from build123d import *

# Parameters (mm, degrees)
F1_DEPTH = 31.75
F2_R     = 12.7
F4_DEPTH = 76.201


with BuildPart() as f1:
    # F0 (on Front) → F1 (new body)
    with BuildSketch(Plane.XZ):
        with BuildLine():
            ThreePointArc((-73.025, 0), (0, 73.025), (73.025, 0))
            Line((73.025, 0), (73.025, -73.025))
            Line((73.025, -73.025), (76.2, -73.025))
            Line((76.2, -73.025), (76.2, 0))
            ThreePointArc((76.2, 0), (0, 76.2), (-76.2, 0))
            Line((-76.2, 0), (-76.2, -73.025))
            Line((-76.2, -73.025), (-73.025, -73.025))
            Line((-73.025, -73.025), (-73.025, 0))
        make_face()
    extrude(amount=F1_DEPTH)

    # F2
    f2_edges = [f1.edges().sort_by_distance(p)[0] for p in [
        (-74.6125, -31.75, -73.025),
        (-74.6125, 0, -73.025),
        (74.6125, -31.75, -73.025),
        (74.6125, 0, -73.025),
    ]]
    fillet(f2_edges, radius=F2_R)

    # F3 (on Top) → F4 (cut, through all)
    with BuildSketch(Plane.XY):
        with BuildLine():
            ThreePointArc((-69.85, -17.4625), (-68.920064, -19.707564), (-66.675, -20.6375))
            Line((-66.675, -20.6375), (66.675, -20.6375))
            ThreePointArc((66.675, -20.6375), (68.920064, -19.707564), (69.85, -17.4625))
            Line((69.85, -17.4625), (69.85, -14.2875))
            ThreePointArc((69.85, -14.2875), (68.920064, -12.042436), (66.675, -11.1125))
            Line((66.675, -11.1125), (-66.675, -11.1125))
            ThreePointArc((-66.675, -11.1125), (-68.920064, -12.042436), (-69.85, -14.2875))
            Line((-69.85, -14.2875), (-69.85, -17.4625))
        make_face()
    extrude(amount=F4_DEPTH, mode=Mode.SUBTRACT)


solid = f1.part
Geometry: final body of the model. Coordinates: model frame, mm. A direction names the side the tool comes from. Give positions to 0.01 mm unless a question says otherwise; leave off trailing zeros. Loops run counter-clockwise (first coordinate to the right, second up) from the corner with the lowest first, then second, coordinate; pieces in that order, holes last. Notation, with made-up numbers: (44.5, -21) - (71.5, -21) arc R14 ccw to (71.5, 2) - close; hole circle Ø3 at (36, -10). An arc over 180 degrees is marked (long way). Answer as CSV lines item,"result". Start each with the question number.
1. Section D-D, the plane y = -2.5. Return loops of the section in (x, z) (3 decimals), plus the area to 3 significant figures.
2. Draft query along X for faces 1 (the face through (73.025, -16, -36)), 2 (the face through (1.68, -8.6, 76.18)), 3 (the face through (-74.59, -27.931, -69.403)). Return one class per face: released by +X, released by -X, zero draft, split by the parting line, or undercut.
3. Ray query, L1, parallel to X at y = -19.5, z = -18 (3 decimals); L2, parallel to Z at x = -1.5, y = -30; L3, parallel to X at y = -14.5, z = 5. Return the intervals inside material, ascending.
4. Section B-B, the plane z = -23. Return loops of the section in (x, y) (3 decimals), plus the area to 3 significant figures.
5. Reachability of faces 4 (the face through (74.635, -3.819, -69.403)), 5 (the face through (-73.025, -16, -37)) from +Z, -Z, +X, -X, +Y, -Y: full face, straight path, thin tool, end or side. Return the list, or none.
6. Section C-C, the plane z = 46. Return loops of the section in (x, y), plus the area to 3 significant figures.
7. Pin query (flat end, axial travel): P1, Ø3.5, axis at y = -16.5, z = 23.5, coming from the +X side; P2, Ø1, axis at x = 29, y = -8, coming from the -Z side; P3, Ø6, axis at x = -8, y = -9.5, coming from the +Z side. Return the tip coordinate at first contact, or that it passes through.
Answers:
1,outline,"(-76.2, -67.891) - (-73.025, -67.891) - (-73.025, 0) arc R73.025 cw to (73.025, 0) - (73.025, -67.891) - (76.2, -67.891) - (76.2, 0) arc R76.2 ccw to (-76.2, 0) - close"
1,area,"1,180 mm2"
2,face 1,"undercut"
2,face 2,"split by the parting line"
2,face 3,"zero draft"
3,L1,"x = -76.2 to -73.025, 73.025 to 76.2"
3,L2,"z = 73.01 to 76.19"
3,L3,"x = -76.04 to -72.85, 72.85 to 76.04"
4,outline,"(-76.2, -31.75) - (-73.025, -31.75) - (-73.025, 0) - (-76.2, 0) - close; (73.025, -31.75) - (76.2, -31.75) - (76.2, 0) - (73.025, 0) - close"
4,area,"202 mm2"
5,face 4,"-Z, +X, -X, +Y"
5,face 5,"-Z, +Y, -Y"
6,outline,"(-60.75, -31.75) - (-56.72, -31.75) - (-56.72, -20.64) - (-60.75, -20.64) - close; (-60.75, -11.11) - (-56.72, -11.11) - (-56.72, 0) - (-60.75, 0) - close; (56.72, -31.75) - (60.75, -31.75) - (60.75, -20.64) - (56.72, -20.64) - close; (56.72, -11.11) - (60.75, -11.11) - (60.75, 0) - (56.72, 0) - close"
6,area,"179 mm2"
7,P1,"stops at x = 73.03"
7,P2,"stops at z = 66.8"
7,P3,"stops at z = 76.04"
